```python
from build123d import *

# Parameters (mm, degrees)
SKETCH1_R                                = 6
SKETCH1_R_2                              = 2
ARDUINO_OFFSET_PINS_DEPTH                = 10
ARDUINO_OFFSET_PINS_2_DEPTH              = 10
ARDUINO_OFFSET_PINS_3_DEPTH              = 10
ARDUINO_OFFSET_PINS_4_DEPTH              = 10
SKETCH2_W                                = 160
SKETCH2_H                                = 65
SKETCH2_R                                = 2
BATTERY_HOLDER_BASE_DEPTH                = 3
SKETCH3_R                                = 4
BATTERY_HOLDER_ARDUINO_COUNTERSINK_DEPTH = 3
BATTERYHOLDER_WALLS_DEPTH                = 25
SEEED_HOLDER_WALLS_DEPTH                 = 25
SEEED_HOLDER_CAP_DEPTH                   = 3


with BuildPart() as part:
    # Sketch1 → Arduino Offset Pins (new body)
    with BuildSketch(Plane(origin=(0, 0, 0), x_dir=(1, 0, 0), z_dir=(0, 1, 0))):
        with Locations(Location((0, 28, 0), (0, 0, 270))):
            Circle(SKETCH1_R)
        with Locations(Location((0, 28, 0), (0, 0, 270))):
            Circle(SKETCH1_R_2, mode=Mode.SUBTRACT)
    extrude(amount=ARDUINO_OFFSET_PINS_DEPTH)



with BuildPart() as body_2:
    # Sketch1 → Arduino Offset Pins 2 (new body)
    with BuildSketch(Plane(origin=(0, 0, 0), x_dir=(1, 0, 0), z_dir=(0, 1, 0))):
        with Locations(Location((0, 0, 0), (0, 0, 270))):
            Circle(SKETCH1_R)
        with Locations(Location((0, 0, 0), (0, 0, 270))):
            Circle(SKETCH1_R_2, mode=Mode.SUBTRACT)
    extrude(amount=ARDUINO_OFFSET_PINS_2_DEPTH)


with BuildPart() as body_3:
    # Sketch1 → Arduino Offset Pins 3 (new body)
    with BuildSketch(Plane(origin=(0, 0, 0), x_dir=(1, 0, 0), z_dir=(0, 1, 0))):
        with Locations(Location((52, -5, 0), (0, 0, 270))):
            Circle(SKETCH1_R)
        with Locations(Location((52, -5, 0), (0, 0, 270))):
            Circle(SKETCH1_R_2, mode=Mode.SUBTRACT)
    extrude(amount=ARDUINO_OFFSET_PINS_3_DEPTH)


with BuildPart() as body_4:
    # Sketch1 → Arduino Offset Pins 4 (new body)
    with BuildSketch(Plane(origin=(0, 0, 0), x_dir=(1, 0, 0), z_dir=(0, 1, 0))):
        with Locations(Location((50, 43, 0), (0, 0, 270))):
            Circle(SKETCH1_R)
        with Locations(Location((50, 43, 0), (0, 0, 270))):
            Circle(SKETCH1_R_2, mode=Mode.SUBTRACT)
    extrude(amount=ARDUINO_OFFSET_PINS_4_DEPTH)


with BuildPart() as part_1:
    add(part.part)

    add(body_2.part)  # battery holder base merges body 2

    add(body_3.part)  # battery holder base merges body 3

    add(body_4.part)  # battery holder base merges body 4
    # Sketch2 → battery holder base (add)
    with BuildSketch(Plane(origin=(0, 10, 0), x_dir=(1, 0, 0), z_dir=(0, 1, 0))):
        with Locations((17.5, 19)):
            Rectangle(SKETCH2_W, SKETCH2_H)
        with Locations(Location((0, 0, 0), (0, 0, 270))):
            Circle(SKETCH2_R, mode=Mode.SUBTRACT)
        with Locations(Location((0, 28, 0), (0, 0, 270))):
            Circle(SKETCH2_R, mode=Mode.SUBTRACT)
        with Locations(Location((50, 43, 0), (0, 0, 270))):
            Circle(SKETCH2_R, mode=Mode.SUBTRACT)
        with Locations(Location((52, -5, 0), (0, 0, 270))):
            Circle(SKETCH2_R, mode=Mode.SUBTRACT)
    extrude(amount=BATTERY_HOLDER_BASE_DEPTH)

    # Sketch3 → Battery Holder Arduino Countersink (cut)
    with BuildSketch(Plane(origin=(0, 13, 0), x_dir=(1, 0, 0), z_dir=(0, 1, 0))):
        with Locations(Location((0, 0, 0), (0, 0, 270))):
            Circle(SKETCH3_R)
        with Locations(Location((0, 28, 0), (0, 0, 270))):
            Circle(SKETCH3_R)
        with Locations(Location((52, -5, 0), (0, 0, 270))):
            Circle(SKETCH3_R)
        with Locations(Location((50, 43, 0), (0, 0, 270))):
            Circle(SKETCH3_R)
    extrude(amount=-BATTERY_HOLDER_ARDUINO_COUNTERSINK_DEPTH, mode=Mode.SUBTRACT)

    # Sketch4 → BatteryHolder Walls (add)
    with BuildSketch(Plane(origin=(0, 13, 0), x_dir=(1, 0, 0), z_dir=(0, 1, 0))):
        Polygon((-62.5, -13.5), (97.5, -13.5), (97.5, -8.5), (-57.5, -8.5), (-57.5, 46.5), (97.5, 46.5), (97.5, 51.5), (-62.5, 51.5), (-62.5, 46.5), (-62.5, -8.5), align=None)
    extrude(amount=BATTERYHOLDER_WALLS_DEPTH)

    # Sketch6 → SEEED holder walls (add)
    with BuildSketch(Plane.XZ.offset(-10)):
        Polygon((-34.5, -32), (-34.5, -6), (-62.5, -6), (-62.5, -9), (-37.5, -9), (-37.5, -29), (-62.5, -29), (-62.5, -32), align=None)
        Polygon((-43.5, -19), (-43.5, -15.658875471), (-46.5, -15.658875471), (-46.5, -19), (-46.5, -22.341124529), (-43.5, -22.341124529), align=None)
    extrude(amount=SEEED_HOLDER_WALLS_DEPTH)

    # Sketch7 → Seeed holder cap (add)
    with BuildSketch(Plane.XZ.offset(15)):
        Polygon((-48.5, -15.658875471), (-48.5, -6), (-62.5, -6), (-62.5, -32), (-48.5, -32), (-48.5, -22.341124529), (-43.5, -22.341124529), (-43.5, -15.658875471), align=None)
    extrude(amount=SEEED_HOLDER_CAP_DEPTH)


solid = part_1.part
```
Design review of the part built by this model. Coordinates are the model's own, in mm. A direction names the side the tool comes from. Give positions to 0.01 mm unless a question says otherwise; leave off trailing zeros. Write each loop counter-clockwise with the first axis right and the second up, starting at its lowest first coordinate (ties: lowest second). Pieces come first, ordered by that corner, then holes. Notation, with made-up numbers: (-34, 28.25) - (23, 28.25) arc R18 ccw to (23, 50.25) - close; hole circle Ø5 at (-30, -20). An arc over 180 degrees is marked (long way). Return JSON: item names as keys, results as strings. Group by question number.
(1) We need section B-B, the plane z = -43. Give the boundary of the cut face in (x, y).
(2) Machinability: for faces 4 (the flat face through (-34.5, -2, -19)), 5 (the flat face through (21, 25, 8.5)), 6 (the flat face through (-50, -2, -9)), 7 (the flat face through (-49, -4, -32)), which of the approach directions +Z, -Z, +X, -X, +Y, -Y give a long, thin tool a straight path to every point of the face, cutting with its end or side? Answer none if there is none.
(3) Mouldability with a two-part tool opening along Y and no side actions: class faces 1 (the flat face through (49, 0, 5)), 2 (the flat face through (-1, 10, -2)), 3 (the flat face through (-55, -15, -19)) as +Y half, -Y half, draft (parallel to the pull), parting line (faces both ways), or undercut.
(4) To check wall thickness, follow probe 1 along X at (y, z) = (4, -28); probe 2 along Z at (x, y) = (39.5, 22); probe 3 along X at (y, z) = (12.15, 0). State the ranges of each line that lie inside material, in increasing order.
(5) We need section C-C, the plane x = -23. Give the boundary of the cut face in (y, z), then the cut area to 3 significant figures.
(6) We need section D-D, the plane y = 17. Give the boundary of the cut face in (x, z).
(7) We need section A-A, the plane y = 4. Give the number of separate pieces and of enclosed holes in the cut face, then the cut area to 3 significant figures.
(8) Insertion check: pin 1 (5.5 mm diameter, centred on y = 3.5, z = -19.5, fed in from -X); pin 2 (4 mm diameter, centred on x = -1, z = -1.5, fed in from +Y); pin 3 (1 mm diameter, centred on x = -7.5, z = -34, fed in from +Y); pin 4 (6.5 mm diameter, centred on x = 51.5, z = 5.5, fed in from +Y). Each pin has a flat end and moves straight along its axis. Give the tip position at first contact, or say it passes through.
Reported:
{
 "1": {"outline": "(-62.5, 10) - (44, 10) - (44, 0) - (48, 0) - (48, 10) - (46, 10) - (46, 13) - (-57.5, 13) - (-57.5, 38) - (-62.5, 38) - close; (52, 0) - (56, 0) - (56, 10) - (97.5, 10) - (97.5, 13) - (54, 13) - (54, 10) - (52, 10) - close"},
 "2": {"face 4": "+Z, -Z, -Y", "face 5": "+X, +Y", "face 6": "-X", "face 7": "-Z, -X, -Y"},
 "3": {"face 1": "-Y half", "face 2": "+Y half", "face 3": "undercut"},
 "4": {"probe 1": "x = -37.5 to -34.5, -6 to -2, 2 to 6", "probe 2": "z = -51.5 to -46.5, 8.5 to 13.5", "probe 3": "x = -62.5 to -4, 4 to 97.5"},
 "5": {"outline": "(10, -51.5) - (38, -51.5) - (38, -46.5) - (13, -46.5) - (13, 8.5) - (38, 8.5) - (38, 13.5) - (10, 13.5) - close", "area": "445 mm2"},
 "6": {"outline": "(-62.5, -51.5) - (97.5, -51.5) - (97.5, -46.5) - (-57.5, -46.5) - (-57.5, 8.5) - (97.5, 8.5) - (97.5, 13.5) - (-62.5, 13.5) - close"},
 "7": {"separate pieces": "6", "enclosed holes": "4", "area": "650 mm2"},
 "8": {"pin 1": "stops at x = -46.5", "pin 2": "stops at y = 10", "pin 3": "stops at y = 13", "pin 4": "stops at y = 38"}
}
